from build123d import *
from build123d.topology import SkipClean

# Parameters (mm, degrees)
SKETCH1_R                   = 13.75
MOTOR_BODY_DEPTH            = 32.5
SKETCH7_R                   = 5
MOTOR_TIP_DEPTH             = 3
SKETCH8_W                   = 3
SKETCH8_H                   = 0.75
MOTOR_CONTACTS_DEPTH        = 6.5
MOTOR_CONTACTS_CHAMFER_SIZE = 0.75
MOTOR_CONTACTS_HOLE_DEPTH   = 23.25
CONNECTION_BOT_1_DEPTH      = 3
SKETCH14_R                  = 19.25
CONNECTION_BOT_2_DEPTH      = 1
SKETCH10_R                  = 18.5
CONNECTION_MID_DEPTH        = 15
CONNECTION_TOP_1_DEPTH      = 3
CONNECTION_TOP_2_START      = 1
SKETCH12_R                  = 3.5
CONNECTION_TOP_2_DEPTH      = 1
SKETCH13_R                  = 2.5
SCREW_HOLDERS_DEPTH         = 15
SKETCH3_R                   = 1.5
SCREW_HOLES_DEPTH           = 22
SKETCH15_R                  = 6
SKETCH15_R_2                = 4.125
MOTOR_SHAFT_GUIDE_DEPTH     = 5
SKETCH16_R                  = 4
MOTOR_SHAFT_BOT_DEPTH       = 4
MOTOR_SHAFT_DEPTH           = 9


with BuildPart() as part:
    # Sketch1 → motor_body (new body)
    with BuildSketch(Plane(origin=(0, 0, 0), x_dir=(1, 0, 0), z_dir=(0, 1, 0))):
        with Locations(Location((0, 0, 0), (0, 0, 270))):
            Circle(SKETCH1_R)
    extrude(amount=MOTOR_BODY_DEPTH)

    # Sketch7 → motor_tip (add)
    with BuildSketch(Plane.XZ):
        with Locations(Location((0, 0, 0), (0, 0, 270))):
            Circle(SKETCH7_R)
    extrude(amount=MOTOR_TIP_DEPTH)

    # Sketch8 → motor_contacts (add)
    with BuildSketch(Plane.XZ):
        with Locations((0, 11.625)):
            Rectangle(SKETCH8_W, SKETCH8_H)
        with Locations((0, -11.625)):
            Rectangle(SKETCH8_W, SKETCH8_H)
    extrude(amount=MOTOR_CONTACTS_DEPTH)

    # motor_contacts_chamfer
    motor_contacts_chamfer_edges = [part.edges().sort_by_distance(p)[0] for p in [
        (1.5, -6.5, 11.625),
        (-1.5, -6.5, 11.625),
        (-1.5, -6.5, -11.625),
        (1.5, -6.5, -11.625),
    ]]
    chamfer(motor_contacts_chamfer_edges, length=MOTOR_CONTACTS_CHAMFER_SIZE)

    # Sketch9 → motor_contacts_hole (cut)
    with BuildSketch(Plane.XY.offset(12)):
        with BuildLine():
            Line((0.79375, -3.79375), (0.79375, -4.70625))
            ThreePointArc((0.79375, -4.70625), (0, -5.5), (-0.79375, -4.70625))
            Line((-0.79375, -4.70625), (-0.79375, -3.79375))
            ThreePointArc((-0.79375, -3.79375), (0, -3), (0.79375, -3.79375))
        make_face()
    motor_contacts_hole = extrude(amount=-MOTOR_CONTACTS_HOLE_DEPTH, mode=Mode.SUBTRACT)

    # motor_contacts_hole2: motor_contacts_hole across plane
    add(motor_contacts_hole.mirror(Plane.XY), mode=Mode.SUBTRACT)

    # Sketch2 → connection_bot_1 (add)
    with BuildSketch(Plane(origin=(0, 32.5, 0), x_dir=(1, 0, 0), z_dir=(0, 1, 0))):
        with BuildLine():
            Line((19.181980515, 12.818019485), (16.416641448, 10.052680417))
            ThreePointArc((16.416641448, 10.052680417), (19.24991098, -0.058542722), (16.355194034, -10.152345941))
            Line((16.355194034, -10.152345941), (19.181980515, -12.818019485))
            ThreePointArc((19.181980515, -12.818019485), (19.181980515, -19.181980515), (12.818019485, -19.181980515))
            Line((12.818019485, -19.181980515), (10.052680417, -16.416641448))
            ThreePointArc((10.052680417, -16.416641448), (-0.058542722, -19.24991098), (-10.152345941, -16.355194034))
            Line((-10.152345941, -16.355194034), (-12.818019485, -19.181980515))
            ThreePointArc((-12.818019485, -19.181980515), (-19.181980515, -19.181980515), (-19.181980515, -12.818019485))
            Line((-19.181980515, -12.818019485), (-16.416641448, -10.052680417))
            ThreePointArc((-16.416641448, -10.052680417), (-19.24991098, 0.058542722), (-16.355194034, 10.152345941))
            Line((-16.355194034, 10.152345941), (-19.181980515, 12.818019485))
            ThreePointArc((-19.181980515, 12.818019485), (-19.181980515, 19.181980515), (-12.818019485, 19.181980515))
            Line((-12.818019485, 19.181980515), (-10.052680417, 16.416641448))
            ThreePointArc((-10.052680417, 16.416641448), (0.058542722, 19.24991098), (10.152345941, 16.355194034))
            Line((10.152345941, 16.355194034), (12.818019485, 19.181980515))
            ThreePointArc((12.818019485, 19.181980515), (19.181980515, 19.181980515), (19.181980515, 12.818019485))
        make_face()
    extrude(amount=CONNECTION_BOT_1_DEPTH)

    # Sketch14 → connection_bot_2 (add)
    with BuildSketch(Plane(origin=(0, 35.5, 0), x_dir=(1, 0, 0), z_dir=(0, 1, 0))):
        with Locations(Location((0, 0, 0), (0, 0, 121.48109236))):
            Circle(SKETCH14_R)
    extrude(amount=CONNECTION_BOT_2_DEPTH)

    # Sketch10 → connection_mid (add)
    with BuildSketch(Plane(origin=(0, 36.5, 0), x_dir=(1, 0, 0), z_dir=(0, 1, 0))):
        with Locations(Location((0, 0, 0), (0, 0, 270))):
            Circle(SKETCH10_R)
    extrude(amount=CONNECTION_MID_DEPTH)

    # Sketch11 → connection_top_1 (add)
    with SkipClean():  # the faces are left unmerged after this step: merging them gives an invalid solid
        with BuildSketch(Plane(origin=(0, 51.5, 0), x_dir=(1, 0, 0), z_dir=(0, 1, 0))):
            with BuildLine():
                Line((-16, 19.5), (16, 19.5))
                ThreePointArc((16, 19.5), (18.474873734, 18.474873734), (19.5, 16))
                Line((19.5, 16), (19.5, -16))
                ThreePointArc((19.5, -16), (18.474873734, -18.474873734), (16, -19.5))
                Line((16, -19.5), (-16, -19.5))
                ThreePointArc((-16, -19.5), (-18.474873734, -18.474873734), (-19.5, -16))
                Line((-19.5, -16), (-19.5, 16))
                ThreePointArc((-19.5, 16), (-18.474873734, 18.474873734), (-16, 19.5))
            make_face()
        extrude(amount=CONNECTION_TOP_1_DEPTH)

    # Sketch12 → connection_top_2 (add)
    with SkipClean():  # the faces are left unmerged after this step: merging them gives an invalid solid
        with BuildSketch(Plane.XZ.offset(-51.5).offset(CONNECTION_TOP_2_START)):
            with Locations(Location((-16, 16, 0), (0, 0, 270))):
                Circle(SKETCH12_R)
            with Locations(Location((16, 16, 0), (0, 0, 270))):
                Circle(SKETCH12_R)
            with Locations(Location((16, -16, 0), (0, 0, 270))):
                Circle(SKETCH12_R)
            with Locations(Location((-16, -16, 0), (0, 0, 270))):
                Circle(SKETCH12_R)
        extrude(amount=-CONNECTION_TOP_2_DEPTH)

    # Sketch13 → screw_holders (add)
    with SkipClean():  # the faces are left unmerged after this step: merging them gives an invalid solid
        with BuildSketch(Plane(origin=(0, 35.5, 0), x_dir=(1, 0, 0), z_dir=(0, 1, 0))):
            with Locations(Location((-16, -16, 0), (0, 0, 90))):
                Circle(SKETCH13_R)
            with Locations(Location((-16, 16, 0), (0, 0, 90))):
                Circle(SKETCH13_R)
            with Locations(Location((16, 16, 0), (0, 0, 90))):
                Circle(SKETCH13_R)
            with Locations(Location((16, -16, 0), (0, 0, 90))):
                Circle(SKETCH13_R)
        extrude(amount=SCREW_HOLDERS_DEPTH)

    # Sketch3 → screw_holes (cut)
    with SkipClean():  # the faces are left unmerged after this step: merging them gives an invalid solid
        with BuildSketch(Plane(origin=(0, 54.5, 0), x_dir=(1, 0, 0), z_dir=(0, 1, 0))):
            with Locations(Location((-16, 16, 0), (0, 0, 270))):
                Circle(SKETCH3_R)
            with Locations(Location((16, 16, 0), (0, 0, 270))):
                Circle(SKETCH3_R)
            with Locations(Location((16, -16, 0), (0, 0, 270))):
                Circle(SKETCH3_R)
            with Locations(Location((-16, -16, 0), (0, 0, 270))):
                Circle(SKETCH3_R)
        extrude(amount=-SCREW_HOLES_DEPTH, mode=Mode.SUBTRACT)

    # Sketch15 → motor_shaft_guide (add)
    with SkipClean():  # the faces are left unmerged after this step: merging them gives an invalid solid
        with BuildSketch(Plane(origin=(0, 54.5, 0), x_dir=(1, 0, 0), z_dir=(0, 1, 0))):
            with Locations(Location((0, 0, 0), (0, 0, 270))):
                Circle(SKETCH15_R)
            with Locations(Location((0, 0, 0), (0, 0, 270))):
                Circle(SKETCH15_R_2, mode=Mode.SUBTRACT)
        extrude(amount=MOTOR_SHAFT_GUIDE_DEPTH)

    # Sketch16 → motor_shaft_bot (add)
    with SkipClean():  # the faces are left unmerged after this step: merging them gives an invalid solid
        with BuildSketch(Plane(origin=(0, 54.5, 0), x_dir=(1, 0, 0), z_dir=(0, 1, 0))):
            with Locations(Location((0, 0, 0), (0, 0, 270))):
                Circle(SKETCH16_R)
        extrude(amount=MOTOR_SHAFT_BOT_DEPTH)

    # Sketch17 → motor_shaft (add)
    with SkipClean():  # the faces are left unmerged after this step: merging them gives an invalid solid
        with BuildSketch(Plane(origin=(0, 58.5, 0), x_dir=(1, 0, 0), z_dir=(0, 1, 0))):
            with BuildLine():
                Line((-1, -1), (-1, -3.872983346))
                ThreePointArc((-1, -3.872983346), (0, -4), (1, -3.872983346))
                Line((1, -3.872983346), (1, -1))
                Line((1, -1), (3.872983346, -1))
                ThreePointArc((3.872983346, -1), (4, 0), (3.872983346, 1))
                Line((3.872983346, 1), (1, 1))
                Line((1, 1), (1, 3.872983346))
                ThreePointArc((1, 3.872983346), (0, 4), (-1, 3.872983346))
                Line((-1, 3.872983346), (-1, 1))
                Line((-1, 1), (-3.872983346, 1))
                ThreePointArc((-3.872983346, 1), (-4, 0), (-3.872983346, -1))
                Line((-3.872983346, -1), (-1, -1))
            make_face()
        extrude(amount=MOTOR_SHAFT_DEPTH)


solid = part.part
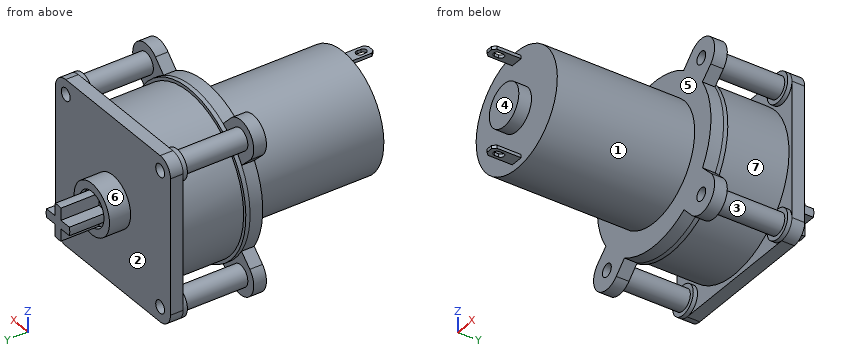
The model under review builds one solid part; all positions refer to its coordinate system, in mm. Face numbers are marked on the shaded views. A direction names the side the tool comes from. Give positions to 0.01 mm unless a question says otherwise; leave off trailing zeros. Write each loop counter-clockwise with the first axis right and the second up, starting at its lowest first coordinate (ties: lowest second). Pieces come first, ordered by that corner, then holes. Notation, with made-up numbers: M -6.5,42 L 36.5,42 A31 ccw 36.5,74 Z; hole C 59,41 d10. An arc over 180 degrees is marked long. One line per question, with ' | ' between items. Start each with the question number.
Item 1: For the marked faces 1, 2, 3 and 4, list the 3-axis set-ups (+Z, -Z, +X, -X, +Y, -Y) from which the entire face can be reached by the end or side of a thin tool; tool diameter is ignored.
Item 2: We need section B-B on y = 18.5. Write out the cut boundary in (x, z), plus the area to 3 significant figures.
Item 3: Draft analysis for pull direction Z (two halves, no side actions). For the marked faces 5, 6 and 7, state which applies: released by +Z, released by -Z, zero draft, split by the parting line, or undercut.
Item 4: We need section D-D on z = 8.5. Write out the cut boundary in (x, y).
Item 5: We need section C-C on x = -8. Write out the cut boundary in (y, z), plus the area to 3 significant figures.
Item 6: Wall thickness on line 1 (X direction, y = 53, z = 16); line 2 (Y direction, x = -16.5, z = 8.5); line 3 (X direction, y = 42, z = -16): over which ranges is each line inside the solid? List them lowest first. Write a range as from..to.
Item 7: For pin 1 (3 mm diameter, centred on y = 64, z = 2, fed in from -X); pin 2 (12 mm diameter, centred on x = -3.5, y = 9, fed in from +Z); pin 3 (13 mm diameter, centred on x = 0, z = 0, fed in from -Y); pin 4 (2.5 mm diameter, centred on x = -16, z = 16, fed in from +Y), all flat-tipped, find the tip position at first contact; note any pin that passes through.
Results found:
1) face 1: -Y | face 2: +Y | face 3: none | face 4: +X, -X, -Y
2) outline: C 0,0 d27.5 | area: 594 mm2
3) face 5: zero draft | face 6: split by the parting line | face 7: undercut
4) outline: M -19.5,51.5 L -16.43,51.5 L -16.43,36.5 L -17.27,36.5 L -17.27,32.5 L -10.81,32.5 L -10.81,0 L 10.81,0 L 10.81,32.5 L 17.27,32.5 L 17.27,36.5 L 16.43,36.5 L 16.43,51.5 L 19.5,51.5 L 19.5,54.5 L -19.5,54.5 Z
5) outline: M 0,-11.18 L 32.5,-11.18 L 32.5,-17.51 L 36.5,-17.51 L 36.5,-16.68 L 51.5,-16.68 L 51.5,-19.5 L 54.5,-19.5 L 54.5,19.5 L 51.5,19.5 L 51.5,16.68 L 36.5,16.68 L 36.5,17.51 L 32.5,17.51 L 32.5,11.18 L 0,11.18 Z | area: 1,480 mm2
6) line 1: x = -19.5..-17.5, -14.5..14.5, 17.5..19.5 | line 2: y = 32.5..36.5, 51.5..54.5 | line 3: x = -18.5..-17.5, -14.5..-13.5, -9.29..9.29, 13.5..14.5, 17.5..18.5
7) pin 1: stops at x = -3.97 | pin 2: stops at z = 13.75 | pin 3: stops at y = -3 | pin 4: passes through
